Geometry check sheet. Reference: the model listing, model coordinates, mm. A direction names the side the tool comes from. Round coordinates to 2 decimals unless told otherwise and drop trailing zeros. Write each loop counter-clockwise with the first axis right and the second up, starting at its lowest first coordinate (ties: lowest second). Pieces come first, ordered by that corner, then holes. Notation, with made-up numbers: M 35,81.25 L 53,81.25 A25 ccw 53,96.25 Z; hole C 63,44.25 d7. An arc over 180 degrees is marked long. Answer as CSV lines item,"result". Start each with the question number.
```python
from build123d import *

# Parameters (mm, degrees)
SKETCH1_W           = 130
SKETCH1_H           = 60
BOSS_EXTRUDE1_DEPTH = 12
CUT_EXTRUDE1_START  = -5
SKETCH2_W           = 22
SKETCH2_H           = 10
CUT_EXTRUDE1_DEPTH  = 129.955216397
CUT_EXTRUDE2_START  = -2
SKETCH3_W           = 0.6
SKETCH3_H           = 8.4
SKETCH3_H_2         = 0.6
SKETCH3_W_2         = 17.05
CUT_EXTRUDE2_DEPTH  = 1
CUT_EXTRUDE3_START  = -2
SKETCH3_3_W         = 17.05
SKETCH3_3_H         = 8.4
CUT_EXTRUDE3_DEPTH  = 2
BOSS_EXTRUDE2_DEPTH = 80
FILLET1_R           = 0.4
FILLET2_R           = 1


with BuildPart() as part:
    # Sketch1 → Boss-Extrude1 (new body)
    with BuildSketch(Plane(origin=(0, 0, 0), x_dir=(1, 0, 0), z_dir=(0, 1, 0))):
        Rectangle(SKETCH1_W, SKETCH1_H)
    extrude(amount=BOSS_EXTRUDE1_DEPTH)

    # Sketch2 → Cut-Extrude1 (cut, through all)
    with BuildSketch(Plane(origin=(65, 0, 0), x_dir=(0, 0, -1), z_dir=(1, 0, 0)).offset(CUT_EXTRUDE1_START)):
        with Locations((15, 7)):
            Rectangle(SKETCH2_W, SKETCH2_H)
    cut_extrude1 = extrude(amount=-CUT_EXTRUDE1_DEPTH, mode=Mode.SUBTRACT)

    # Mirror1: Cut-Extrude1 across plane
    add(cut_extrude1.mirror(Plane.XY), mode=Mode.SUBTRACT)

    # Sketch3 → Cut-Extrude2 (cut)
    with BuildSketch(Plane.ZY.offset(-60).offset(CUT_EXTRUDE2_START)):
        with Locations((23.825, 7.8)):
            Rectangle(SKETCH3_W, SKETCH3_H)
        with Locations((23.825, 3.3)):
            Rectangle(SKETCH3_W, SKETCH3_H_2)
        with Locations((15, 7.8)):
            Rectangle(SKETCH3_W_2, SKETCH3_H)
        with Locations((15, 3.3)):
            Rectangle(SKETCH3_W_2, SKETCH3_H_2)
        with Locations((6.175, 3.3)):
            Rectangle(SKETCH3_W, SKETCH3_H_2)
        with Locations((6.175, 7.8)):
            Rectangle(SKETCH3_W, SKETCH3_H)
    cut_extrude2 = extrude(amount=CUT_EXTRUDE2_DEPTH, mode=Mode.SUBTRACT)

    # Sketch3<3> → Cut-Extrude3 (cut)
    with BuildSketch(Plane.ZY.offset(-60).offset(CUT_EXTRUDE3_START)):
        with Locations((15, 7.8)):
            Rectangle(SKETCH3_3_W, SKETCH3_3_H)
    cut_extrude3 = extrude(amount=CUT_EXTRUDE3_DEPTH, mode=Mode.SUBTRACT)

    # Mirror2: Cut-Extrude2, Cut-Extrude3 across plane
    add(cut_extrude2.mirror(Plane.XY), mode=Mode.SUBTRACT)
    add(cut_extrude3.mirror(Plane.XY), mode=Mode.SUBTRACT)

    # Sketch4 → Boss-Extrude2 (add)
    with BuildSketch(Plane.ZY.offset(65)):
        Polygon((4, 2), (4, 8.5), (1.75, 8.5), (1.75, 6.5), (-1.75, 6.5), (-1.75, 8.5), (-4, 8.5), (-4, 2), (-4, 0), (4, 0), align=None)
    extrude(amount=BOSS_EXTRUDE2_DEPTH)

    # Fillet1
    fillet1_edges = [part.edges().sort_by_distance(p)[0] for p in [
        (-105, 8.5, -1.75),
        (-105, 8.5, -4),
        (-145, 4.25, 4),
        (-105, 8.5, 4),
        (-105, 8.5, 1.75),
        (-145, 4.25, -4),
    ]]
    fillet(fillet1_edges, radius=FILLET1_R)

    # Fillet2
    fillet2_edges = [part.edges().sort_by_distance(p)[0] for p in [
        (0, 12, 30),
        (-2.5, 12, -4),
        (-2.5, 12, -26),
        (-2.5, 12, 26),
        (-2.5, 12, 4),
        (65, 6, 30),
        (-65, 6, 30),
        (-65, 6, -30),
        (65, 6, -30),
        (0, 12, -30),
    ]]
    fillet(fillet2_edges, radius=FILLET2_R)


solid = part.part
```
1) Go/stop test with flat-tipped pins: pin 1 (11 mm diameter, centred on x = -26.5, z = 19, fed in from +Y); pin 2 (1.5 mm diameter, centred on y = 10.5, z = -6, fed in from -X); pin 3 (0.5 mm diameter, centred on x = 60.5, z = 11, fed in from +Y). Record where each tip stops, or that it passes through.
2) Section check A-A, the plane z = 11. Record the cut outline in (x, y), plus the area to 3 significant figures.
3) Mould release check, pull along Z, two halves, no side actions. Record for faces 1 (the flat face through (-65, 1, -20)), 2 (the flat face through (-65, 10, 0)), 3 (the flat face through (60, 3, 15)): released by +Z, released by -Z, zero draft, split by the parting line, or undercut.
4) Scan lines: line 1 (Z direction, x = 18.5, y = 9.25); line 2 (Z direction, x = -94.5, y = 7.25); line 3 (X direction, y = 3.5, z = 7.5). Record each from-to range of solid material in increasing order. Write a range as from..to.
5) Section check B-B, the plane x = 26. Record the cut outline in (y, z).
6) Access from +Z, -Z, +X, -X, +Y, -Y to the whole of each face (thin tool, end or side, straight path). Record for faces 4 (the flat face through (61, 3.2, 14.3)), 5 (the flat face through (-65, 1.5, 20.3)), 6 (the flat face through (60, 3, -15)).
7) Section check C-C, the plane x = -87. Record the cut outline in (y, z), plus the area to 3 significant figures.
Results:
1,pin 1,"stops at y = 2"
1,pin 2,"stops at x = 60"
1,pin 3,"stops at y = 3.6"
2,outline,"M -65,0 L 65,0 L 65,12 L 62,12 L 62,3 L 61,3 L 61,3.6 L 60,3.6 L 60,2 L -65,2 Z"
2,area,"293 mm^2"
3,face 1,"zero draft"
3,face 2,"undercut"
3,face 3,"undercut"
4,line 1,"z = -30..-26, -4..4, 26..30"
4,line 2,"z = -4..-1.75, 1.75..4"
4,line 3,"x = 60..61, 62..65"
5,outline,"M 0,-30 L 11,-30 A1 ccw 12,-29 L 12,-27 A1 ccw 11,-26 L 2,-26 L 2,-4 L 11,-4 A1 ccw 12,-3 L 12,3 A1 ccw 11,4 L 2,4 L 2,26 L 11,26 A1 ccw 12,27 L 12,29 A1 ccw 11,30 L 0,30 Z"
6,face 4,"+Y"
6,face 5,"+Z, -X, +Y, -Y"
6,face 6,"-X, +Y"
7,outline,"M 0,-4 L 8.1,-4 A0.4 ccw 8.5,-3.6 L 8.5,-2.15 A0.4 ccw 8.1,-1.75 L 6.5,-1.75 L 6.5,1.75 L 8.1,1.75 A0.4 ccw 8.5,2.15 L 8.5,3.6 A0.4 ccw 8.1,4 L 0,4 Z"
7,area,"60.9 mm^2"
